Here's how the part is built. I have some questions about the finished solid (model axes, mm). Face numbers are marked on the shaded views. A direction names the side the tool comes from. Round coordinates to 2 decimals unless told otherwise and drop trailing zeros. Write each loop counter-clockwise with the first axis right and the second up, starting at its lowest first coordinate (ties: lowest second). Pieces come first, ordered by that corner, then holes. Notation, with made-up numbers: (29, 73.25) -> (86, 73.25) arc R17 ccw to (86, 96.25) -> close; hole circle Ø4 at (-24.75, 39.25). An arc over 180 degrees is marked (long way). Answer as CSV lines item,"result".
```python
from build123d import *

# Parameters (mm, degrees)
BOSS_EXTRUDE1_DEPTH = 14
CUT_EXTRUDE1_DEPTH  = 3.2
SKETCH4_W           = 0.4
SKETCH4_H           = 1
CUT_EXTRUDE3_DEPTH  = 17.414932226
BOSS_EXTRUDE2_START = -3.2
BOSS_EXTRUDE2_DEPTH = 0.6
SKETCH3_R           = 2.125
CUT_EXTRUDE2_DEPTH  = 16.966292619


with BuildPart() as part:
    # Sketch1 → Boss-Extrude1 (new body)
    with BuildSketch(Plane(origin=(0, 0, 0), x_dir=(1, 0, 0), z_dir=(0, 1, 0))):
        with BuildLine():
            Line((-3.509834179, 2.212636718), (-5.25, 0.254950169))
            Line((-5.25, 0.254950169), (-5.25, -1))
            Line((-5.25, -1), (-2.85, -1))
            Line((-2.85, -1), (-2.85, -2.8))
            Line((-2.85, -2.8), (2.85, -2.8))
            Line((2.85, -2.8), (2.85, -1))
            Line((2.85, -1), (5.25, -1))
            Line((5.25, -1), (5.25, 0.254950169))
            Line((5.25, 0.254950169), (3.509834179, 2.212636718))
            ThreePointArc((3.509834179, 2.212636718), (2.918765962, 2.646420098), (2.201867871, 2.8))
            Line((2.201867871, 2.8), (-2.201867871, 2.8))
            ThreePointArc((-2.201867871, 2.8), (-2.918765962, 2.646420098), (-3.509834179, 2.212636718))
        make_face()
    extrude(amount=BOSS_EXTRUDE1_DEPTH)

    # Sketch2 → Cut-Extrude1 (cut)
    with BuildSketch(Plane(origin=(0, 0, -2.8), x_dir=(-1, 0, 0), z_dir=(0, 0, -1))):
        Polygon((-3.55, 4.950406544), (0, 2.900813089), (3.55, 4.950406544), (3.55, 9.049593456), (0, 11.099186911), (-3.55, 9.049593456), align=None)
    extrude(amount=-CUT_EXTRUDE1_DEPTH, mode=Mode.SUBTRACT)

    # Sketch4 → Cut-Extrude3 (cut, through all)
    with BuildSketch(Plane.ZY.offset(2.85)):
        with Locations((0.8, 12)):
            Rectangle(SKETCH4_W, SKETCH4_H)
        with Locations((0.8, 10)):
            Rectangle(SKETCH4_W, SKETCH4_H)
        with Locations((0.8, 8)):
            Rectangle(SKETCH4_W, SKETCH4_H)
        with Locations((0.8, 6)):
            Rectangle(SKETCH4_W, SKETCH4_H)
        with Locations((0.8, 4)):
            Rectangle(SKETCH4_W, SKETCH4_H)
        with Locations((0.8, 2)):
            Rectangle(SKETCH4_W, SKETCH4_H)
    cut_extrude3 = extrude(amount=CUT_EXTRUDE3_DEPTH, mode=Mode.SUBTRACT)

    # Mirror1: Cut-Extrude3 across plane
    add(cut_extrude3.mirror(Plane(origin=(0, 0, 0), x_dir=(0, 0, 1), z_dir=(1, 0, 0))), mode=Mode.SUBTRACT)

    # Sketch2<2> → Boss-Extrude2 (add)
    with BuildSketch(Plane(origin=(0, 0, -2.8), x_dir=(-1, 0, 0), z_dir=(0, 0, -1)).offset(BOSS_EXTRUDE2_START)):
        Polygon((-3.55, 4.950406544), (0, 2.900813089), (3.55, 4.950406544), (3.55, 9.049593456), (0, 11.099186911), (-3.55, 9.049593456), align=None)
    extrude(amount=-BOSS_EXTRUDE2_DEPTH)

    # Sketch3 → Cut-Extrude2 (cut, through all)
    with BuildSketch(Plane.XY.offset(2.8)):
        with Locations((0, 7)):
            Circle(SKETCH3_R)
    extrude(amount=-CUT_EXTRUDE2_DEPTH, mode=Mode.SUBTRACT)


solid = part.part
```
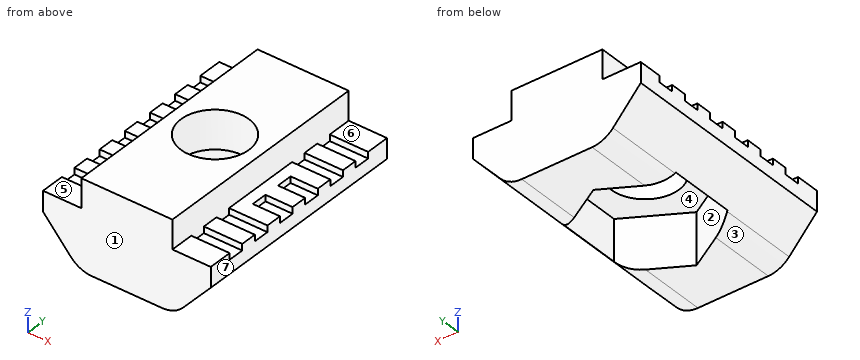
1. Suppose I cut it at D-D on x = -4. Please give me the cut outline in (y, z).
Numbers:
outline,"(0, -1.66) -> (14, -1.66) -> (14, 1) -> (12.5, 1) -> (12.5, 0.6) -> (11.5, 0.6) -> (11.5, 1) -> (10.5, 1) -> (10.5, 0.6) -> (9.5, 0.6) -> (9.5, 1) -> (8.5, 1) -> (8.5, 0.6) -> (7.5, 0.6) -> (7.5, 1) -> (6.5, 1) -> (6.5, 0.6) -> (5.5, 0.6) -> (5.5, 1) -> (4.5, 1) -> (4.5, 0.6) -> (3.5, 0.6) -> (3.5, 1) -> (2.5, 1) -> (2.5, 0.6) -> (1.5, 0.6) -> (1.5, 1) -> (0, 1) -> close"
2. On a 3-axis mill with a long thin cutter (end or side, diameter ignored), from which of +Z, -Z, +X, -X, +Y, -Y can I reach the whole of each face in a straight line? I mean the marked faces 4, 5, 6 and 7. Say none if no direction works.
Numbers:
face 4,"-Z"
face 5,"+Z, -X, +Y, -Y"
face 6,"+Z, +X, +Y, -Y"
face 7,"+Z, -Z, +X, +Y, -Y"
3. Suppose I cut it at A-A on y = 7. Please give me the cut outline in (x, z) (3 decimals), and give its area (3 significant figures).
Numbers:
outline,"(-5.25, -0.255) -> (-3.55, -2.167) -> (-3.55, 0.4) -> (-2.125, 0.4) -> (-2.125, 2.8) -> (-2.85, 2.8) -> (-2.85, 1) -> (-5.25, 1) -> close; (2.125, 0.4) -> (3.55, 0.4) -> (3.55, -2.167) -> (5.25, -0.255) -> (5.25, 1) -> (2.85, 1) -> (2.85, 2.8) -> (2.125, 2.8) -> close"
area,"11.8 mm^2"
4. Suppose I cut it at C-C on y = 2. Please give me the cut outline in (x, z).
Numbers:
outline,"(-5.25, -0.25) -> (-3.51, -2.21) arc R1.75 ccw to (-2.2, -2.8) -> (2.2, -2.8) arc R1.75 ccw to (3.51, -2.21) -> (5.25, -0.25) -> (5.25, 0.6) -> (2.85, 0.6) -> (2.85, 2.8) -> (-2.85, 2.8) -> (-2.85, 0.6) -> (-5.25, 0.6) -> close"
5. If we mould it in two halves opening along X, with no side actions, what happens to the marked faces 1, 2 and 3? For each: released by +X, released by -X, zero draft, split by the parting line, or undercut.
Numbers:
face 1,"zero draft"
face 2,"undercut"
face 3,"released by -X"
6. If I drill on line 1 (Y direction, x = 0, z = 1.1) (3 decimals); line 2 (Z direction, x = 0.5, y = 9.75); line 3 (X direction, y = 5.75, z = 0), over which ranges is the centre line in solid material (lowest first)?
Numbers:
line 1,"y = 0 to 4.875, 9.125 to 14"
line 2,"z = 0.4 to 2.8"
line 3,"x = -5.25 to -3.55, 3.55 to 5.25"
7. For pin 1 Ø0.5 at (x, y) = (4.5, 3) entering from +Z; pin 2 Ø0.8 at (x, y) = (-4.5, 8) entering from +Z, each with a flat end and sliding along its axis, tell me the tip position at first contact or that it passes through.
Numbers:
pin 1,"stops at z = 1"
pin 2,"stops at z = 0.6"
8. Suppose I cut it at B-B on z = -1.55. Please give me the cut outline in (x, y).
Numbers:
outline,"(-4.1, 0) -> (4.1, 0) -> (4.1, 14) -> (-4.1, 14) -> close; hole (-3.55, 4.95) -> (0, 2.9) -> (3.55, 4.95) -> (3.55, 9.05) -> (0, 11.1) -> (-3.55, 9.05) -> close"
